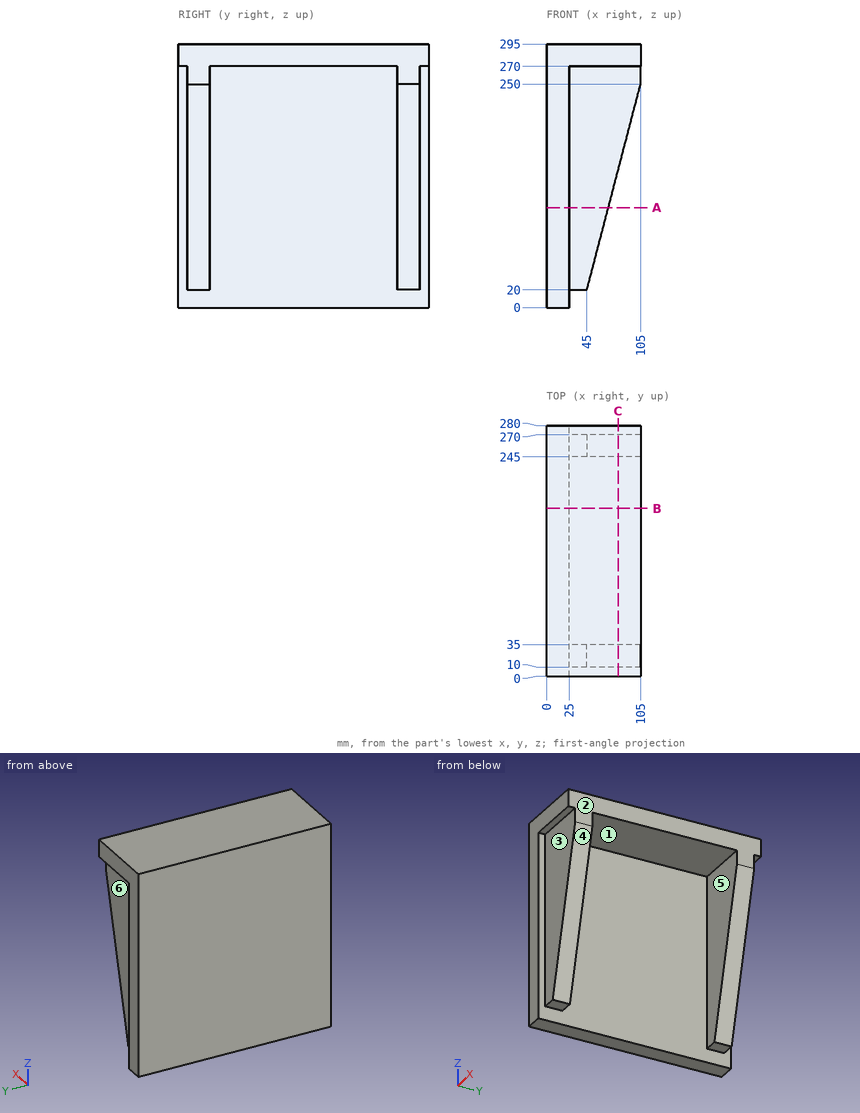
The figure shows three views and two pictorial views of one solid part (mm, origin at its lowest corner). Answer the questions. A direction names the side the tool comes from. Give positions to 0.01 mm unless a question says otherwise; leave off trailing zeros. Order: outer loops, then holes, each group sorted by start corner. A loop starts at its lowest first (then second) coordinate and runs counter-clockwise, first axis right, second up. Notation, with made-up numbers: M -3,-23 L 49,-23 A30 cw 49,4 Z; hole C 37,-33.5 d9. An arc over 180 degrees is marked long. Return JSON: item names as keys, results as strings.
Q1. Find the intervals of material crossed by line 1 along Y through (x, z) = (52.5, 168); line 2 along X through (y, z) = (182, 206.5); line 3 along Z through (x, y) = (58, 138.5), in increasing order. Write a range as [from, to].
Answer below:
{"line 1": "y = [10, 35], [245, 270]", "line 2": "x = [0, 25]", "line 3": "z = [270, 295]"}
Q2. Each of these flat-tipped pins is pushed along its axis until it touches: pin 1 (6 mm diameter, centred on x = 68.5, y = 100.5, fed in from -Z); pin 2 (6 mm diameter, centred on x = 34.5, y = 28.5, fed in from -Z); pin 3 (16 mm diameter, centred on x = 30, y = 254, fed in from -Z); pin 4 (6 mm diameter, centred on x = 47.5, z = 245, fed in from -Y). Where does it stop, or does it pass through?
Answer below:
{"pin 1": "stops at z = 270", "pin 2": "stops at z = 20", "pin 3": "stops at z = 0", "pin 4": "stops at y = 10"}
Q3. Find section A-A, the plane z = 112. Write down the section's boundary in (x, y), and give its area (3 significant figures).
Answer below:
{"outline": "M 0,0 L 25,0 L 25,10 L 69,10 L 69,35 L 25,35 L 25,245 L 69,245 L 69,270 L 25,270 L 25,280 L 0,280 Z", "area": "9,200 mm^2"}
Q4. Find section C-C, the plane x = 80. Write down the section's boundary in (y, z), and give its area (3 significant figures).
Answer below:
{"outline": "M 0,270 L 10,270 L 10,154.17 L 35,154.17 L 35,270 L 245,270 L 245,154.17 L 270,154.17 L 270,270 L 280,270 L 280,295 L 0,295 Z", "area": "12,800 mm^2"}
Q5. The mould has two halves that part along Y. Classify the marked faces 4, 5 and 6: pulls with the +Y half, pulls with the -Y half, needs draft (parallel to the pull), parting line crosses it, or undercut.
Answer below:
{"face 4": "needs draft", "face 5": "undercut", "face 6": "pulls with the +Y half"}
Q6. Find section B-B, the plane y = 187.5. Write down the section's boundary in (x, z), and give its area (4 significant figures).
Answer below:
{"outline": "M 0,0 L 25,0 L 25,270 L 105,270 L 105,295 L 0,295 Z", "area": "9,375 mm^2"}
Q7. Which of the six approach directions +Z, -Z, +X, -X, +Y, -Y give full straight-line access (tool end or side, diameter ignored) to the marked faces 1, 2 and 3?
Answer below:
{"face 1": "-Z, +X", "face 2": "+Z, -Z, +X, +Y, -Y", "face 3": "-Z, +X, -Y"}
